from build123d import *

# Parameters (mm, degrees)
SKETCH1_W           = 2.54
SKETCH1_H           = 1
BASE_EXTRUDE_DEPTH  = 0.381
SKETCH2_W           = 1
SKETCH2_H           = 1
BOSS_EXTRUDE1_DEPTH = 24
SKETCH7_W           = 1
SKETCH7_H           = 1
BOSS_EXTRUDE4_DEPTH = 1
FILLET5_R           = 0.254
BOSS_EXTRUDE2_DEPTH = 1
SKETCH4_R           = 2.5
BOSS_EXTRUDE3_DEPTH = 7.6
FILLET4_R           = 2.5
SKETCH6_W           = 0.032
SKETCH6_H           = 0.381
CUT_EXTRUDE1_DEPTH  = 4.45


with BuildPart() as part:
    # Sketch1 → Base-Extrude (new body)
    with BuildSketch(Plane(origin=(0, 0, 0), x_dir=(1, 0, 0), z_dir=(0, 1, 0))):
        with Locations((0.77, 0)):
            Rectangle(SKETCH1_W, SKETCH1_H)
    extrude(amount=BASE_EXTRUDE_DEPTH)

    # Sketch2 → Boss-Extrude1 (add)
    with BuildSketch(Plane.XZ):
        Rectangle(SKETCH2_W, SKETCH2_H)
        with Locations((1.54, 0)):
            Rectangle(SKETCH2_W, SKETCH2_H)
    extrude(amount=BOSS_EXTRUDE1_DEPTH)

    # Sketch7 → Boss-Extrude4 (add)
    with BuildSketch(Plane.XZ.offset(24)):
        Rectangle(SKETCH7_W, SKETCH7_H)
    extrude(amount=BOSS_EXTRUDE4_DEPTH)

    # Fillet5
    fillet5_edges = [part.edges().sort_by_distance(p)[0] for p in [
        (2.04, 0.381, 0),
        (0.5, 0, 0),
        (1.04, 0, 0),
        (-0.5, 0.381, 0),
    ]]
    fillet(fillet5_edges, radius=FILLET5_R)

    # Sketch3 → Boss-Extrude2 (add)
    with BuildSketch(Plane(origin=(0, 0.381, 0), x_dir=(-1, 0, 0), z_dir=(0, 1, 0))):
        with BuildLine():
            Line((-2.336045976, 2.5), (0.796045976, 2.5))
            ThreePointArc((0.796045976, 2.5), (-0.77, -2.95), (-2.336045976, 2.5))
        make_face()
    extrude(amount=BOSS_EXTRUDE2_DEPTH)

    # Sketch4 → Boss-Extrude3 (add)
    with BuildSketch(Plane(origin=(0, 1.381, 0), x_dir=(-1, 0, 0), z_dir=(0, 1, 0))):
        with Locations((-0.77, 0)):
            Circle(SKETCH4_R)
    extrude(amount=BOSS_EXTRUDE3_DEPTH)

    # Fillet4
    fillet4_edges = [part.edges().sort_by_distance(p)[0] for p in [
        (3.27, 8.981, 0),
    ]]
    fillet(fillet4_edges, radius=FILLET4_R)

    # Sketch6 → Cut-Extrude1 (cut, through all)
    with BuildSketch(Plane.XY.offset(0.5)):
        with Locations((0.77, 0.1905)):
            Rectangle(SKETCH6_W, SKETCH6_H)
    extrude(amount=-CUT_EXTRUDE1_DEPTH, mode=Mode.SUBTRACT)


solid = part.part
Geometry check sheet. Reference: the model listing, model coordinates, mm. A direction names the side the tool comes from. Coordinates: 2 decimals unless noted, no trailing zeros. Order: outer loops, then holes, each group sorted by start corner. A loop starts at its lowest first (then second) coordinate and runs counter-clockwise, first axis right, second up. Notation, with made-up numbers: (-28.75, -30) -> (16.25, -30) arc R27 cw to (16.25, -6) -> close; hole circle Ø5 at (-35, 29). An arc over 180 degrees is marked (long way). Use a Markdown table: item, result. Add a question column.
1. Mould release check, pull along X, two halves, no side actions. Record for faces 1 (the face through (1.31, 3.9, -2.44)), 2 (the face through (0, -12, -0.5)), 3 (the face through (0.5, -12, 0)): pulls with the +X half, pulls with the -X half, needs draft (parallel to the pull), parting line crosses it, or undercut.
2. Cross-section at C-C (x = -1.2). Enter the section's corners in (y, z).
3. Cross-section at D-D (y = 4.5). Enter the section's corners in (x, z), and give its area (3 significant figures).
4. Set-up check for faces 4 (the face through (1.5, -24, 0)), 5 (the face through (0, -12, 0.5)), 6 (the face through (-0.5, -12, 0)), 7 (the face through (1.04, -12, 0)): record each of +Z, -Z, +X, -X, +Y, -Y from which the full face is reachable in a straight line by a thin tool's end or side.
5. Go/stop test with flat-tipped pins: pin 1 Ø0.5 at (y, z) = (-16.5, 0) entering from +X; pin 2 Ø2 at (x, z) = (-0.5, -2) entering from -Y; pin 3 Ø0.6 at (x, y) = (0, -13) entering from -Z. Record where each tip stops, or that it passes through.
6. Material ranges on L1, parallel to X at y = -3.5, z = -0.1; L2, parallel to Z at x = -0.35, y = 0; L3, parallel to Y at x = 1.2, z = 2.25, recorded low to high.
7. Cross-section at A-A (y = -22). Enter the section's corners in (x, z), and give its area (3 significant figures).
Filled sheet:
| question | item | result |
|---|---|---|
| 1 | face 1 | parting line crosses it |
| 1 | face 2 | needs draft |
| 1 | face 3 | undercut |
| 2 | outline | (0.38, -2.2) -> (1.38, -2.2) -> (1.38, -1.54) -> (6.48, -1.54) arc R1.54 ccw to (6.48, 1.54) -> (1.38, 1.54) -> (1.38, 2.2) -> (0.38, 2.2) -> close |
| 3 | outline | circle Ø5 at (0.77, 0) |
| 3 | area | 19.6 mm2 |
| 4 | face 4 | +Z, -Z, +X, -Y |
| 4 | face 5 | +Z, +X, -X, -Y |
| 4 | face 6 | +Z, -Z, -X, -Y |
| 4 | face 7 | +Z, -Z, -Y |
| 5 | pin 1 | x = 2.04 |
| 5 | pin 2 | y = 0.38 |
| 5 | pin 3 | z = -0.5 |
| 6 | L1 | -0.5 to 0.5, 1.04 to 2.04 |
| 6 | L2 | -0.5 to 0.5 |
| 6 | L3 | 0.38 to 7.48 |
| 7 | outline | (-0.5, -0.5) -> (0.5, -0.5) -> (0.5, 0.5) -> (-0.5, 0.5) -> close; (1.04, -0.5) -> (2.04, -0.5) -> (2.04, 0.5) -> (1.04, 0.5) -> close |
| 7 | area | 2.00 mm2 |
